The listing builds one solid part. Answer for the finished solid, in the listing's coordinates (mm). A direction names the side the tool comes from. Coordinates: 2 decimals unless noted, no trailing zeros. Write each loop counter-clockwise with the first axis right and the second up, starting at its lowest first coordinate (ties: lowest second). Pieces come first, ordered by that corner, then holes.
(1) The part is cut by section C-C on z = 1.75. Determine the outline of the cut face in (x, y), plus the area to 3 significant figures.
(2) Straight lines are drawn through the part: line 1 (Y direction, x = 33.75, z = 4); line 2 (X direction, y = -11.75, z = 6.25); line 3 (Y direction, x = 0, z = 0.6). For each, find the intervals that lie inside material, in ascending order.
(3) Which of the six approach directions +Z, -Z, +X, -X, +Y, -Y give full straight-line access (tool end or side, diameter ignored) to faces 1 (the flat face through (0, -10, 1)), 2 (the cylindrical face through (-38.039, 8.196, 1.479)), 3 (the cylindrical face through (28.755, -11.78, 5.465))?
(4) Given P1, Ø6, axis at x = 0, y = 0, coming from the +Z side; P2, Ø2.5, axis at x = 8, z = 1.5, coming from the -Y side, each flat-ended and moving along its own axis, determine where each tip first touches the part or whether it passes through.
(5) For a pull along X with two mould halves and no side action, classify faces 4 (the flat face through (-31.6, -11.9, 8)), 5 (the cylindrical face through (37.946, 8.289, 1.479)), 6 (the cylindrical face through (35.4, -11.93, 3.94)) as +X half, -X half, draft (parallel to the pull), parting line (faces both ways), or undercut.
(6) The part is cut by section D-D on z = 6.25. Determine the outline of the cut face in (x, y).
(7) The part is cut by section A-A on y = 0. Determine the outline of the cut face in (x, z), plus the area to 3 significant figures.
(8) The part is cut by section B-B on x = 0. Determine the outline of the cut face in (y, z).
from build123d import *

# Parameters (mm, degrees)
EXTRUDE_1_DEPTH    = 3
SKETCH_4_R         = 5
EXTRUDE_2_DEPTH    = 5
M4X0_7_1_D         = 3.3
HOLE_WIZARD_M4_1_D = 4.5


with BuildPart() as part:
    # 草圖1 → 填料-伸長1 (new body)
    with BuildSketch(Plane.XY):
        with BuildLine():
            Line((-33.75, 10), (33.75, 10))
            ThreePointArc((33.75, 10), (37.992640687, 8.242640687), (39.75, 4))
            Line((39.75, 4), (39.75, -12))
            ThreePointArc((39.75, -12), (33.75, -18), (27.75, -12))
            ThreePointArc((27.75, -12), (27.164213562, -10.585786438), (25.75, -10))
            Line((25.75, -10), (-25.75, -10))
            ThreePointArc((-25.75, -10), (-27.164213562, -10.585786438), (-27.75, -12))
            ThreePointArc((-27.75, -12), (-33.75, -18), (-39.75, -12))
            Line((-39.75, -12), (-39.75, 4))
            ThreePointArc((-39.75, 4), (-37.992640687, 8.242640687), (-33.75, 10))
        make_face()
    extrude(amount=EXTRUDE_1_DEPTH)

    # 草圖4 → 填料-伸長2 (add)
    with BuildSketch(Plane.XY.offset(3)):
        with Locations((-33.75, -12)):
            Circle(SKETCH_4_R)
        with Locations((33.75, -12)):
            Circle(SKETCH_4_R)
    extrude(amount=EXTRUDE_2_DEPTH)

    # M4x0.7 螺紋孔1 (through all)
    with Locations(Plane.XY.offset(8)):
        with Locations((-33.75, -12), (33.75, -12)):
            Hole(M4X0_7_1_D / 2)

    # M4 餘隙孔1 (through all)
    with Locations(Plane.XY.offset(3)):
        with Locations((-30, 0), (30, 0), (0, 0)):
            Hole(HOLE_WIZARD_M4_1_D / 2)


solid = part.part
Model answer:
1. outline: (-39.75, -12) arc R6 ccw to (-27.75, -12) arc R2 cw to (-25.75, -10) - (25.75, -10) arc R2 cw to (27.75, -12) arc R6 ccw to (39.75, -12) - (39.75, 4) arc R6 ccw to (33.75, 10) - (-33.75, 10) arc R6 ccw to (-39.75, 4) - close; hole circle Ø3.3 at (-33.75, -12); hole circle Ø4.5 at (-30, 0); hole circle Ø4.5 at (0, 0); hole circle Ø4.5 at (30, 0); hole circle Ø3.3 at (33.75, -12)
1. area: 1,670 mm2
2. line 1: y = -17 to -13.65, -10.35 to -7
2. line 2: x = -38.74 to -35.38, -32.12 to -28.76, 28.76 to 32.12, 35.38 to 38.74
2. line 3: y = -10 to -2.25, 2.25 to 10
3. face 1: +Z, -Z, -Y
3. face 2: +Z, -Z, -X, +Y
3. face 3: +Z
4. P1: stops at z = 3
4. P2: stops at y = -10
5. face 4: draft
5. face 5: +X half
5. face 6: undercut
6. outline: circle Ø10 at (-33.75, -12); circle Ø10 at (33.75, -12); hole circle Ø3.3 at (-33.75, -12); hole circle Ø3.3 at (33.75, -12)
7. outline: (-39.75, 0) - (-32.25, 0) - (-32.25, 3) - (-39.75, 3) - close; (-27.75, 0) - (-2.25, 0) - (-2.25, 3) - (-27.75, 3) - close; (2.25, 0) - (27.75, 0) - (27.75, 3) - (2.25, 3) - close; (32.25, 0) - (39.75, 0) - (39.75, 3) - (32.25, 3) - close
7. area: 198 mm2
8. outline: (-10, 0) - (-2.25, 0) - (-2.25, 3) - (-10, 3) - close; (2.25, 0) - (10, 0) - (10, 3) - (2.25, 3) - close
